Read the model definition and answer for the solid it produces. Units are mm, in the model's axes. A direction names the side the tool comes from. Coordinates: 2 decimals unless noted, no trailing zeros. Write each loop counter-clockwise with the first axis right and the second up, starting at its lowest first coordinate (ties: lowest second). Pieces come first, ordered by that corner, then holes.
1) Find the intervals of material crossed by line 1 (Y direction, x = -86, z = -227); line 2 (Y direction, x = -81, z = -133.5); line 3 (X direction, y = -61.5, z = -112), in increasing order.
2) Each of these flat-tipped pins is pushed along its axis until it touches: pin 1 Ø15 at (y, z) = (-55.5, -86.5) entering from -X; pin 2 Ø3 at (y, z) = (-52.5, 76.5) entering from +X; pin 3 Ø10 at (y, z) = (-49.5, 103.5) entering from -X. Where does it stop, or does it pass through?
3) The part is cut by section C-C (z = -113.5). Determine the outline of the cut face in (x, y), then the cut area to 3 significant figures.
4) The part is cut by section A-A (z = -218.5). Determine the outline of the cut face in (x, y), then the cut area to 3 significant figures.
5) Which of the six approach directions +Z, -Z, +X, -X, +Y, -Y give full straight-line access (tool end or side, diameter ignored) to faces 1 (the face through (17.013, -1.426, -93.725)), 2 (the face through (39.093, -44, -227)), 3 (the face through (17.013, -88.574, -93.725)), 4 (the face through (-45, -5, -227)), 5 (the face through (30.36, -44.44, -184.97))?
6) Determine the mould class of faces 6 (the face through (19.58, -44.44, -22.73)), 7 (the face through (-98.37, -88.57, -94.56)), 8 (the face through (-44, -68.506, -108)), 9 (the face through (-45, -18, -191.832)) for opening direction Z: +Z half, -Z half, draft (parallel to the pull), parting line (faces both ways), or undercut.
from build123d import *

# Parameters (mm, degrees)
F1_DEPTH    = 90
F2_T1_DEPTH = 507.1106760185
F2_T3_DEPTH = 372.5735965904
F3_R        = 5
F4_DEPTH    = 70
F5_W        = 86.5122303367
F5_H        = 49.2804106325
F6_DEPTH    = 170


# Not quite as in the source:
# - a fillet or chamfer that OpenCascade refuses, or shapes differently, is made with other operations: its cross-section is extruded or revolved along the edge and cut away or added


with BuildPart() as f1:
    # F0 (on Front) → F1 (new body)
    with BuildSketch(Plane.XZ):
        with BuildLine():
            Line((-126.2623920763, -193.7024648741), (-126.2623920763, -261.8315013925))
            Line((-126.2623920763, -261.8315013925), (39.092946983, -261.8315013925))
            Line((39.092946983, -261.8315013925), (39.092946983, -193.7024648741))
            Line((39.092946983, -193.7024648741), (21.4152774533, -176.0247953445))
            Line((21.4152774533, -176.0247953445), (21.4152774533, -102.6550637093))
            Line((21.4152774533, -102.6550637093), (15.5539703198, -84.1264084333))
            Line((15.5539703198, -84.1264084333), (15.5539703198, -42.2008474989))
            ThreePointArc((15.5539703198, -42.2008474989), (19.6898884351, -22.4740848198), (31.401046165, -6.0698241209))
            Line((31.401046165, -6.0698241209), (185.2309488965, 135.5598457642))
            Line((185.2309488965, 135.5598457642), (-14.4236341973, 305.266241394))
            Line((-14.4236341973, 305.266241394), (-66.2712781132, 297.6301199255))
            Line((-66.2712781132, 297.6301199255), (-11.4975965547, 251.0724906007))
            Line((-11.4975965547, 251.0724906007), (69.4938383905, 182.2297708973))
            Line((69.4938383905, 182.2297708973), (46.0270096541, 154.6217370896))
            Line((46.0270096541, 154.6217370896), (-66.2712781132, 22.5061044222))
            ThreePointArc((-66.2712781132, 22.5061044222), (-83.9215394862, -7.7309119674), (-90.0560672706, -42.2008474989))
            Line((-90.0560672706, -42.2008474989), (-90.0560672706, -84.1264084333))
            Line((-90.0560672706, -84.1264084333), (-108.5847225467, -102.6550637093))
            Line((-108.5847225467, -102.6550637093), (-108.5847225467, -176.0247953445))
            Line((-108.5847225467, -176.0247953445), (-126.2623920763, -193.7024648741))
        make_face()
    extrude(amount=F1_DEPTH)

    # F2: fillet of radius 50 on 2 edges, made by hand

    # F2_s2 → F2_t1 (cut)
    with BuildSketch(Plane.XZ.offset(-208.5553380092)):
        with BuildLine():
            ThreePointArc((-14.4236341973, 305.266241394), (-19.4476593821, 272.3668104124), (-2.7086733301, 243.6019058598))
            Line((-2.7086733301, 243.6019058598), (-66.2712781132, 297.6301199255))
            Line((-66.2712781132, 297.6301199255), (-14.4236341973, 305.266241394))
        make_face()
    extrude(amount=F2_T1_DEPTH, mode=Mode.SUBTRACT)

    # F2_s4 → F2_t3 (cut)
    with BuildSketch(Plane.XZ.offset(-141.2867982952)):
        with BuildLine():
            ThreePointArc((142.1701622159, 172.1615144427), (159.7779231252, 135.0553624638), (143.6543137068, 97.2806489872))
            Line((143.6543137068, 97.2806489872), (185.2309488965, 135.5598457642))
            Line((185.2309488965, 135.5598457642), (142.1701622159, 172.1615144427))
        make_face()
    extrude(amount=F2_T3_DEPTH, mode=Mode.SUBTRACT)

    # F3
    f3_edges = [f1.edges().sort_by_distance(p)[0] for p in [
        (39.092947, -45, -193.702465),
        (21.415277, -45, -176.024795),
        (30.254112, 0, -184.86363),
        (30.254112, -90, -184.86363),
        (-108.584723, 0, -139.33993),
        (-108.584723, -45, -176.024795),
        (-126.262392, -45, -193.702465),
        (-117.423557, 0, -184.86363),
        (-117.423557, -90, -184.86363),
        (-126.262392, -45, -261.831501),
        (-126.262392, 0, -227.766983),
        (-126.262392, -90, -227.766983),
        (-108.584723, -45, -102.655064),
        (-90.056067, -45, -42.200847),
        (-90.056067, -45, -84.126408),
        (-90.056067, 0, -63.163628),
        (-90.056067, -90, -63.163628),
        (-66.271278, -45, 22.506104),
        (-83.921539, 0, -7.730912),
        (-83.921539, -90, -7.730912),
        (63.873264, 0, 238.713878),
        (-14.423634, -45, 305.266241),
        (63.873264, -90, 238.713878),
        (142.170162, -45, 172.161514),
        (39.092947, -45, -261.831501),
        (39.092947, 0, -227.766983),
        (39.092947, -90, -227.766983),
        (-43.584723, 0, -261.831501),
        (1.61128, -90, 102.367938),
        (33.392583, -90, 212.915838),
        (-19.447659, -90, 272.36681),
        (159.777923, -90, 135.055362),
        (87.52768, -90, 45.605412),
        (19.689888, -90, -22.474085),
        (15.55397, -90, -63.163628),
        (18.484624, -90, -93.390736),
        (21.415277, -90, -139.33993),
        (-43.584723, -90, -261.831501),
        (-108.584723, -90, -139.33993),
        (-99.320395, -90, -93.390736),
        (21.415277, -45, -102.655064),
        (15.55397, -45, -84.126408),
        (18.484624, 0, -93.390736),
        (1.61128, 0, 102.367938),
        (159.777923, 0, 135.055362),
        (87.52768, 0, 45.605412),
        (19.689888, 0, -22.474085),
        (15.55397, 0, -63.163628),
        (21.415277, 0, -139.33993),
        (-99.320395, 0, -93.390736),
    ]]
    fillet(f3_edges, radius=F3_R)

    # F4 (cut): a face of the model
    f4_faces = [f1.faces().sort_by_distance(p)[0] for p in [
        (-43.5847225467, -45, -261.8315013925),
    ]]
    extrude(f4_faces, amount=-F4_DEPTH, mode=Mode.SUBTRACT)

    # F5 (on face) → F6 (cut)
    with BuildSketch(Plane(origin=(0, 0, -191.8315013925), x_dir=(1, 0, 0), z_dir=(0, 0, -1))):
        with Locations((-43.2561151683, 43.8658641651)):
            Rectangle(F5_W, F5_H)
    extrude(amount=-F6_DEPTH, mode=Mode.SUBTRACT)


solid = f1.part
Reported:
1. line 1: y = -90 to -85, -5 to 0
1. line 2: y = -90 to -68.51, -19.23 to 0
1. line 3: x = -108.58 to -86.51, 0 to 21.42
2. pin 1: stops at x = -99.93
2. pin 2: stops at x = 122.71
2. pin 3: stops at x = -1.68
3. outline: (-108.58, -85) arc R5 ccw to (-103.58, -90) - (16.42, -90) arc R5 ccw to (21.42, -85) - (21.42, -5) arc R5 ccw to (16.42, 0) - (-103.58, 0) arc R5 ccw to (-108.58, -5) - close; hole (-86.51, -68.51) - (0, -68.51) - (0, -19.23) - (-86.51, -19.23) - close
3. area: 7,420 mm2
4. outline: (-126.26, -85) arc R5 ccw to (-121.26, -90) - (34.09, -90) arc R5 ccw to (39.09, -85) - (39.09, -5) arc R5 ccw to (34.09, 0) - (-121.26, 0) arc R5 ccw to (-126.26, -5) - close; hole (-121.26, -85) - (34.09, -85) - (34.09, -5) - (-121.26, -5) - close
4. area: 2,430 mm2
5. face 1: +X, +Y
5. face 2: -Z, +X, +Y, -Y
5. face 3: +X, -Y
5. face 4: -Z
5. face 5: +X, +Y, -Y
6. face 6: undercut
6. face 7: +Z half
6. face 8: draft
6. face 9: -Z half
